Could you check a few things on this model? Use its own coordinates, in mm. Face numbers are marked on the shaded views. A direction names the side the tool comes from. Coordinates: 2 decimals unless noted, no trailing zeros. Order: outer loops, then holes, each group sorted by start corner. A loop starts at its lowest first (then second) coordinate and runs counter-clockwise, first axis right, second up. Notation, with made-up numbers: (39.25, 30) -> (74.25, 30) arc R21 cw to (74.25, 37) -> close; hole circle Ø1 at (6.5, 87). An arc over 180 degrees is marked (long way). Use a Markdown table: item, result. Add a question column.
1) Thinking about a two-plate mould opening in Z: for the marked faces 4, 5, 6 and 7, which applies, +Z half, -Z half, draft (parallel to the pull), parting line (faces both ways), or undercut?
2) If I drill on L1, parallel to Z at x = 0, y = 5.25; L2, parallel to Y at x = -2, z = -1.75; L3, parallel to X at y = 9.5, z = -2.5, over which ranges is the centre line in solid material (lowest first)? Write a range as [from, to].
3) If we section it at C-C (x = 6.75): Write out the boundary of the cut face in (y, z), plus the area to 3 significant figures.
4) If we section it at A-A (y = 4.25): Write out the boundary of the cut face in (x, z).
5) Which directions (+Z, -Z, +X, -X, +Y, -Y) give clear straight access to the entire face, cutting with the end or side of a thin tool? Please do the marked faces 1, 2 and 3.
6) If we section it at B-B (x = 0): Write out the boundary of the cut face in (y, z), plus the area to 3 significant figures.
7) Will these pins go through, and if not, where does the flat tip stop? pin 1 Ø6 at (x, y) = (6, 7) entering from -Z; pin 2 Ø1.9 at (x, z) = (-1.5, 0) entering from -Y; pin 3 Ø4 at (x, z) = (-2, 0.5) entering from -Y; pin 4 Ø2 at (y, z) = (13.5, -1) entering from -X.
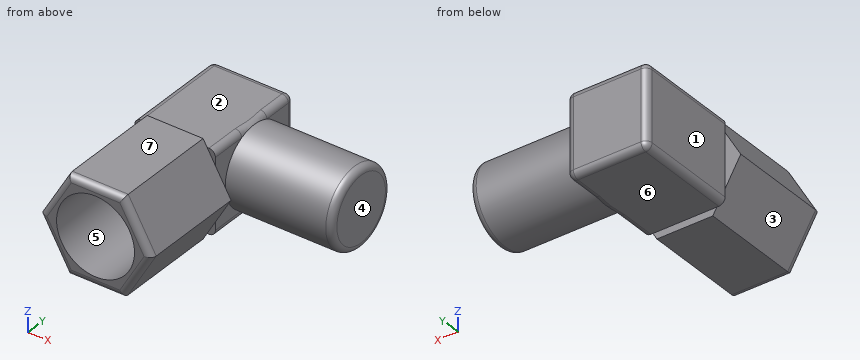
```python
from build123d import *

# Parameters (mm, degrees)
BOSS_EXTRUDE1_DEPTH = 8.5
SKETCH2_W           = 6.4
SKETCH2_H           = 6.6
BOSS_EXTRUDE2_DEPTH = 8.3
SKETCH3_R           = 3.1
BOSS_EXTRUDE3_DEPTH = 8.5
SKETCH4_R           = 3.1
CUT_EXTRUDE1_DEPTH  = 8.5
FILLET1_R           = 0.508


with BuildPart() as part:
    # Sketch1 → Boss-Extrude1 (new body)
    with BuildSketch(Plane(origin=(0, 0, 0), x_dir=(1, 0, 0), z_dir=(0, 1, 0))):
        Polygon((4.445597073, 0), (2.222798536, 3.85), (-2.222798536, 3.85), (-4.445597073, 0), (-2.222798536, -3.85), (2.222798536, -3.85), align=None)
    extrude(amount=BOSS_EXTRUDE1_DEPTH)

    # Sketch2 → Boss-Extrude2 (add)
    with BuildSketch(Plane(origin=(0, 8.5, 0), x_dir=(1, 0, 0), z_dir=(0, 1, 0))):
        Rectangle(SKETCH2_W, SKETCH2_H)
    extrude(amount=BOSS_EXTRUDE2_DEPTH)

    # Sketch3 → Boss-Extrude3 (add)
    with BuildSketch(Plane(origin=(3.2, 0, 0), x_dir=(0, 0, -1), z_dir=(1, 0, 0))):
        with Locations((0, 12.65)):
            Circle(SKETCH3_R)
    extrude(amount=BOSS_EXTRUDE3_DEPTH)

    # Sketch4 → Cut-Extrude1 (cut)
    with BuildSketch(Plane.XZ):
        Circle(SKETCH4_R)
    extrude(amount=-CUT_EXTRUDE1_DEPTH, mode=Mode.SUBTRACT)

    # Fillet1
    fillet1_edges = [part.edges().sort_by_distance(p)[0] for p in [
        (-3.2, 12.65, -3.3),
        (-3.2, 12.65, 3.3),
        (3.2, 12.65, 3.3),
        (3.2, 12.65, -3.3),
        (-3.2, 16.8, 0),
        (0, 16.8, 3.3),
        (3.2, 16.8, 0),
        (0, 16.8, -3.3),
        (11.7, 12.65, 3.1),
        (0, 0, 3.85),
        (-3.334197805, 0, 1.925),
        (-3.334197805, 0, -1.925),
        (0, 0, -3.85),
        (3.334197805, 0, -1.925),
        (3.334197805, 0, 1.925),
    ]]
    fillet(fillet1_edges, radius=FILLET1_R)


solid = part.part
```
Answer sheet:
| question | item | result |
|---|---|---|
| 1 | face 4 | draft |
| 1 | face 5 | undercut |
| 1 | face 6 | -Z half |
| 1 | face 7 | +Z half |
| 2 | L1 | [-3.85, -3.1], [3.1, 3.85] |
| 2 | L2 | [8.5, 16.8] |
| 2 | L3 | [-3.2, 3.2] |
| 3 | outline | circle Ø6.2 at (12.65, 0) |
| 3 | area | 30.2 mm2 |
| 4 | outline | (-4.45, 0) -> (-2.22, -3.85) -> (2.22, -3.85) -> (4.45, 0) -> (2.22, 3.85) -> (-2.22, 3.85) -> close; hole circle Ø6.2 at (0, 0) |
| 5 | face 1 | +Z, -Z, -X, +Y |
| 5 | face 2 | +Z, +X, -X, +Y |
| 5 | face 3 | -Z, -X, -Y |
| 6 | outline | (0, -3.34) arc R0.51 ccw to (0.51, -3.85) -> (8.5, -3.85) -> (8.5, -3.3) -> (16.29, -3.3) arc R0.51 ccw to (16.8, -2.79) -> (16.8, 2.79) arc R0.51 ccw to (16.29, 3.3) -> (8.5, 3.3) -> (8.5, 3.85) -> (0.51, 3.85) arc R0.51 ccw to (0, 3.34) -> (0, 3.1) -> (8.5, 3.1) -> (8.5, -3.1) -> (0, -3.1) -> close |
| 6 | area | 67.3 mm2 |
| 7 | pin 1 | z = -2.5 |
| 7 | pin 2 | y = 8.5 |
| 7 | pin 3 | y = 0 |
| 7 | pin 4 | x = -3.2 |
